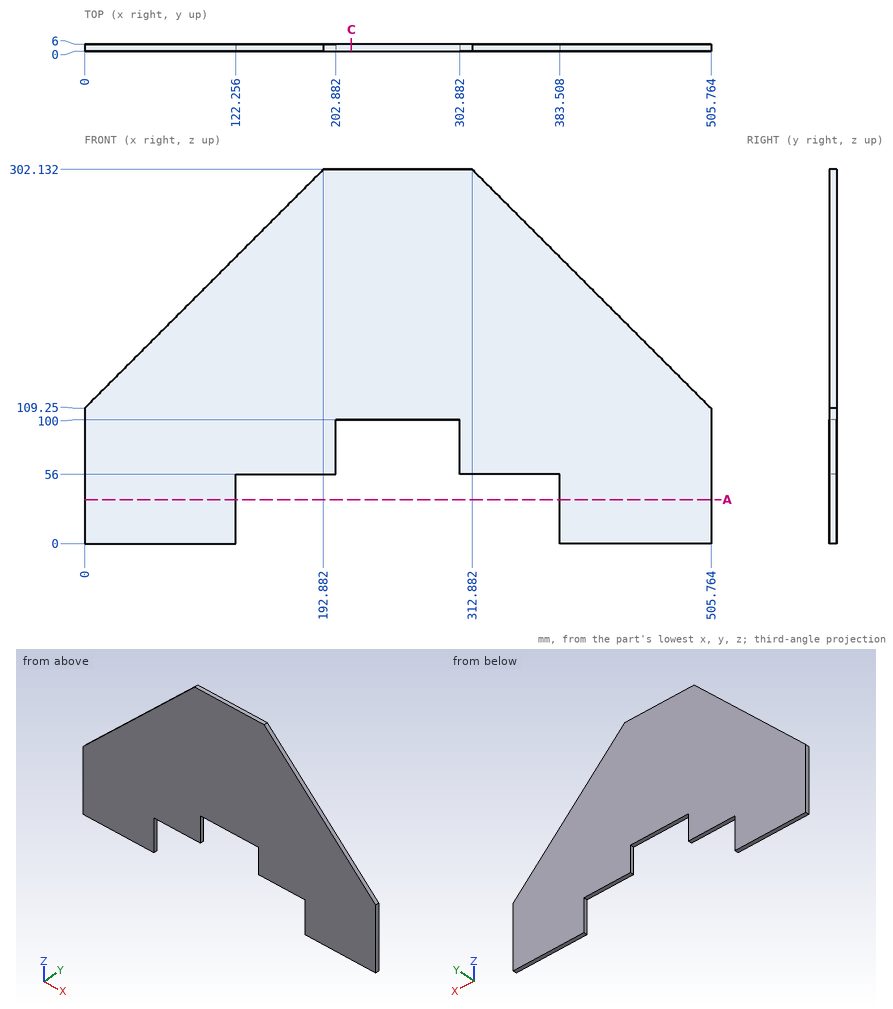
Could you check a few things on this drawing? It's one solid part, dimensions in mm from its lowest x, y, z. Coordinates: 2 decimals unless noted, no trailing zeros. Order: outer loops, then holes, each group sorted by start corner. A loop starts at its lowest first (then second) coordinate and runs counter-clockwise, first axis right, second up. Notation, with made-up numbers: (48.25, 39.5) -> (70.25, 39.5) arc R23 ccw to (70.25, 53.5) -> close; hole circle Ø11 at (20.5, 4.5). An arc over 180 degrees is marked (long way). One line per item, written item: value. Start each with the question number.
1) Imagine slicing it at C-C on x = 215.5. List the corners of the cut face in (y, z) for me, plus the area to 3 significant figures.
2) If I drill on L1, parallel to X at y = 3.65, z = 93 (1 decimal); L2, parallel to X at y = 3.7, z = 15.5 (1 decimal); L3, parallel to Z at x = 270.5, y = 1.7, over which ranges is the centre line in solid material (lowest first)? Write a range as [from, to].
3) Imagine slicing it at A-A on z = 35.5. List the corners of the cut face in (x, y) for me (1 decimal).
4) I'm going to push flat-ended pins straight in: pin 1 (1.8 mm diameter, centred on x = 145.5, y = 3.5, fed in from -Z); pin 2 (1 mm diameter, centred on x = 334.5, y = 2.5, fed in from +Z) (1 decimal). Where does each tip first touch, or does it pass through?
Answer list:
1. outline: (0, 100) -> (6, 100) -> (6, 302.13) -> (0, 302.13) -> close
1. area: 1,210 mm2
2. L1: x = [0, 202.9], [302.9, 505.8]
2. L2: x = [0, 122.3], [383.5, 505.8]
2. L3: z = [100, 302.13]
3. outline: (0, 0) -> (122.3, 0) -> (122.3, 6) -> (0, 6) -> close; (383.5, 0) -> (505.8, 0) -> (505.8, 6) -> (383.5, 6) -> close
4. pin 1: stops at z = 56
4. pin 2: stops at z = 281
